Input: part model. Units: mm. Frame: model coordinates. A direction names the side the tool comes from. Round coordinates to 2 decimals unless told otherwise and drop trailing zeros. Loops run counter-clockwise (first coordinate to the right, second up) from the corner with the lowest first, then second, coordinate; pieces in that order, holes last. Notation, with made-up numbers: (51.5, -37) -> (66.5, -37) arc R19 ccw to (66.5, -30) -> close; hole circle Ø1 at (0, -8.5). An arc over 180 degrees is marked (long way). One line per question, with ' | ' between items. Start each with the question number.
Q1. Contact query for flat-ended pins moving along their axis: P1, Ø3, axis at y = 35.5, z = 1, coming from the -X side; P2, Ø2, axis at x = 24.5, z = 5.5, coming from the -Y side; P3, Ø6, axis at y = 42.5, z = 8, coming from the +X side. Output: stop coordinate, or through.
Q2. Cut plane B-B on y = 30. Return loops of the section in (x, z), and give its area (3 significant figures).
Q3. Cut plane A-A on x = 17. Return loops of the section in (y, z), and give its area (3 significant figures).
Q4. Cut plane C-C on x = -34. Return loops of the section in (y, z).
Q5. Access query for faces 1 (the face through (-39.342, 31, 5)), 2 (the face through (-18.5, 0.07, 4.93)). Directions: +Z, -Z, +X, -X, +Y, -Y. A direction counts if a zero-diameter tool reaches every point of the face in a straight line with its end or side. Return the directions, or none.
Q6. Cut plane D-D on z = 1.25. State how many separate pieces and enclosed holes the cut face has, and give its area (3 significant figures).
Q7. Mould query, pull axis X, two halves, no side actions, for faces 3 (the face through (-9, 1, 0)), 4 (the face through (0, 28, 5)), 5 (the face through (33.939, 49.297, 5.07)), 6 (the face through (-39.342, -31, 5)). Classes: pulls with the +X half, pulls with the -X half, needs draft (parallel to the pull), parting line crosses it, or undercut.
Q8. Material intervals for L1, parallel to X at y = -35, z = 4.75; L2, parallel to Y at x = -34, z = 3.25; L3, parallel to X at y = 36, z = 2.5, sorted ascending.
from build123d import *

# Parameters (mm, degrees)
SKETCH1_R           = 47.5
SKETCH1_R_2         = 2.5
SKETCH1_R_3         = 1.5
BOSS_EXTRUDE1_DEPTH = 10
SKETCH7_W           = 79.294879448
SKETCH7_H           = 30
BOSS_EXTRUDE3_DEPTH = 10
SKETCH3_R           = 2
CUT_EXTRUDE1_DEPTH  = 10
CUT_EXTRUDE2_START  = -10
CUT_EXTRUDE2_DEPTH  = 10
FILLET2_R           = 5
FILLET3_R           = 20
SKETCH8_R           = 2
CUT_EXTRUDE3_DEPTH  = 20


with BuildPart() as part:
    # Sketch1 → Boss-Extrude1 (new body)
    with BuildSketch(Plane.XY):
        Circle(SKETCH1_R)
        Circle(SKETCH1_R_2, mode=Mode.SUBTRACT)
        with Locations((0, 17)):
            Circle(SKETCH1_R_3, mode=Mode.SUBTRACT)
        with Locations((17, 0)):
            Circle(SKETCH1_R_3, mode=Mode.SUBTRACT)
        with Locations((0, -17)):
            Circle(SKETCH1_R_3, mode=Mode.SUBTRACT)
        with Locations((-17, 0)):
            Circle(SKETCH1_R_3, mode=Mode.SUBTRACT)
    extrude(amount=BOSS_EXTRUDE1_DEPTH)

    # Sketch7 → Boss-Extrude3 (add)
    with BuildSketch(Plane(origin=(0, 0, 0), x_dir=(-1, 0, 0), z_dir=(0, 0, -1))):
        with Locations((-0.305848536, 40)):
            Rectangle(SKETCH7_W, SKETCH7_H)
        with Locations((-0.305848536, -40)):
            Rectangle(SKETCH7_W, SKETCH7_H)
    extrude(amount=-BOSS_EXTRUDE3_DEPTH)

    # Sketch3 → Cut-Extrude1 (cut)
    with BuildSketch(Plane.XY.offset(10)):
        with Locations((-34, 35)):
            Circle(SKETCH3_R)
        with Locations((34, 35)):
            Circle(SKETCH3_R)
    cut_extrude1 = extrude(amount=-CUT_EXTRUDE1_DEPTH, mode=Mode.SUBTRACT)

    # Mirror1: Cut-Extrude1 across plane
    add(cut_extrude1.mirror(Plane.ZX), mode=Mode.SUBTRACT)

    # Sketch4 → Cut-Extrude2 (cut)
    with BuildSketch(Plane.XY.offset(10).offset(CUT_EXTRUDE2_START)):
        with BuildLine():
            ThreePointArc((-43.084219849, 20), (-47.5, 0), (-43.084219849, -20))
            ThreePointArc((-43.084219849, -20), (-20, 0), (-43.084219849, 20))
        make_face()
        with BuildLine():
            ThreePointArc((43.084219849, 20), (47.5, 0), (43.084219849, -20))
            ThreePointArc((43.084219849, -20), (20, 0), (43.084219849, 20))
        make_face()
    extrude(amount=CUT_EXTRUDE2_DEPTH, mode=Mode.SUBTRACT)

    # Fillet2
    # the kernel refuses this fillet: 5 mm, written as the material it takes off along each edge
    with BuildSketch(Plane(origin=(43.084219849, -20, -17.522188683), x_dir=(-0.4820770193525399, -0.8761288417876509, 0), z_dir=(0, 0, 1))) as fillet2_piece_1:
        with BuildLine():
            CenterArc((7.965064209, -4.7789061), FILLET2_R, 107.102298128, 89.932791817)
            Line((3.18443662, -6.243692723), (3.088824068, -6.272988455))
            ThreePointArc((3.088824068, -6.272988455), (1.775921643, -3.02815315), (-0.079852724, -0.060195867))
            Line((-0.079852724, -0.060195867), (-0.006836496, 0.099766038))
            ThreePointArc((-0.006836496, 0.099766038), (3.24733545, 0.211131977), (6.465263034, 0.095578122))
            Line((6.465263034, 0.095578122), (6.4946709, 0))
        make_face()
    extrude(amount=45.044377366, mode=Mode.SUBTRACT)
    with BuildSketch(Plane(origin=(43.084219849, 20, -17.522188683), x_dir=(-0.9995074123131517, -0.03138363795144594, 0), z_dir=(0, 0, 1))) as fillet2_piece_2:
        with BuildLine():
            CenterArc((7.876051386, -4.92422643), FILLET2_R, 99.987608256, 89.932791817)
            Line((2.950811143, -5.78562561), (2.852306338, -5.802853594))
            ThreePointArc((2.852306338, -5.802853594), (1.28732359, -2.988739235), (-0.091980358, -0.039237913))
            Line((-0.091980358, -0.039237913), (0.017343518, 0.098484529))
            ThreePointArc((0.017343518, 0.098484529), (3.504437737, -0.206216713), (6.991531955, 0.098484529))
            Line((6.991531955, 0.098484529), (7.008875473, 0))
        make_face()
    extrude(amount=45.044377366, mode=Mode.SUBTRACT)
    with BuildSketch(Plane(origin=(-43.084219849, 20, -19.006257622), x_dir=(0.9993011358017984, -0.037379673423339595, 0), z_dir=(0, 0, 1))) as fillet2_piece_3:
        with BuildLine():
            CenterArc((8.144232965, 4.918935136), FILLET2_R, 158.484077447, 101.184563019)
            Line((3.49265456, 6.752734019), (3.399622992, 6.789409997))
            ThreePointArc((3.399622992, 6.789409997), (1.522188613, 3.492296192), (-0.092214112, 0.038685366))
            Line((-0.092214112, 0.038685366), (0.01793407, -0.098378703))
            ThreePointArc((0.01793407, -0.098378703), (3.623764745, 0.227599929), (7.22959542, -0.098378703))
            Line((7.22959542, -0.098378703), (7.247529489, 0))
        make_face()
    extrude(amount=48.012515244, mode=Mode.SUBTRACT)
    with BuildSketch(Plane(origin=(-43.084219849, -20, -19.006257622), x_dir=(0.4922890050047702, -0.8704318098228104, 0), z_dir=(0, 0, 1))) as fillet2_piece_4:
        with BuildLine():
            CenterArc((8.110651537, 4.97411149), FILLET2_R, 162.982413534, 101.184563019)
            Line((3.329576688, 6.437437594), (3.233955191, 6.466704116))
            ThreePointArc((3.233955191, 6.466704116), (1.866948313, 3.114157454), (-0.079143369, 0.061125503))
            Line((-0.079143369, 0.061125503), (-0.008002635, -0.099679275))
            ThreePointArc((-0.008002635, -0.099679275), (3.801251524, -0.252344442), (7.592340079, -0.09948223))
            Line((7.592340079, -0.09948223), (7.602503049, 0))
        make_face()
    extrude(amount=48.012515244, mode=Mode.SUBTRACT)

    # Fillet3
    fillet3_edges = [part.edges().sort_by_distance(p)[0] for p in [
        (-39.341591188, 55, 5),
        (39.95328826, 55, 5),
        (39.95328826, -55, 5),
        (-39.341591188, -55, 5),
    ]]
    fillet(fillet3_edges, radius=FILLET3_R)

    # Sketch8 → Cut-Extrude3 (cut)
    with BuildSketch(Plane(origin=(0, 0, 0), x_dir=(-1, 0, 0), z_dir=(0, 0, -1))):
        with Locations((0, 30)):
            Circle(SKETCH8_R)
        with Locations((-2, -29.933259094)):
            Circle(SKETCH8_R)
    extrude(amount=-CUT_EXTRUDE3_DEPTH, mode=Mode.SUBTRACT)


solid = part.part
Results:
1) P1: x = -39.34 | P2: y = -54.68 | P3: x = 39.44
2) outline: (-39.34, 0) -> (-2, 0) -> (-2, 10) -> (-39.34, 10) -> close; (2, 0) -> (39.95, 0) -> (39.95, 10) -> (2, 10) -> close | area: 753 mm^2
3) outline: (-55, 0) -> (-1.5, 0) -> (-1.5, 10) -> (-55, 10) -> close; (1.5, 0) -> (55, 0) -> (55, 10) -> (1.5, 10) -> close | area: 1,070 mm^2
4) outline: (-48.61, 0) -> (-37, 0) -> (-37, 10) -> (-48.61, 10) -> close; (-33, 0) -> (-19.23, 0) -> (-19.23, 10) -> (-33, 10) -> close; (19.23, 0) -> (33, 0) -> (33, 10) -> (19.23, 10) -> close; (37, 0) -> (48.61, 0) -> (48.61, 10) -> (37, 10) -> close
5) face 1: +Z, -Z, -X, +Y | face 2: +Z, -Z
6) separate pieces: 1 | enclosed holes: 11 | area: 7,010 mm^2
7) face 3: needs draft | face 4: undercut | face 5: pulls with the +X half | face 6: pulls with the -X half
8) L1: -39.34 to -36, -32 to 32, 36 to 39.95 | L2: -48.61 to -37, -33 to -19.23, 19.23 to 33, 37 to 48.61 | L3: -39.32 to -35.73, -32.27 to 32.27, 35.73 to 39.93
